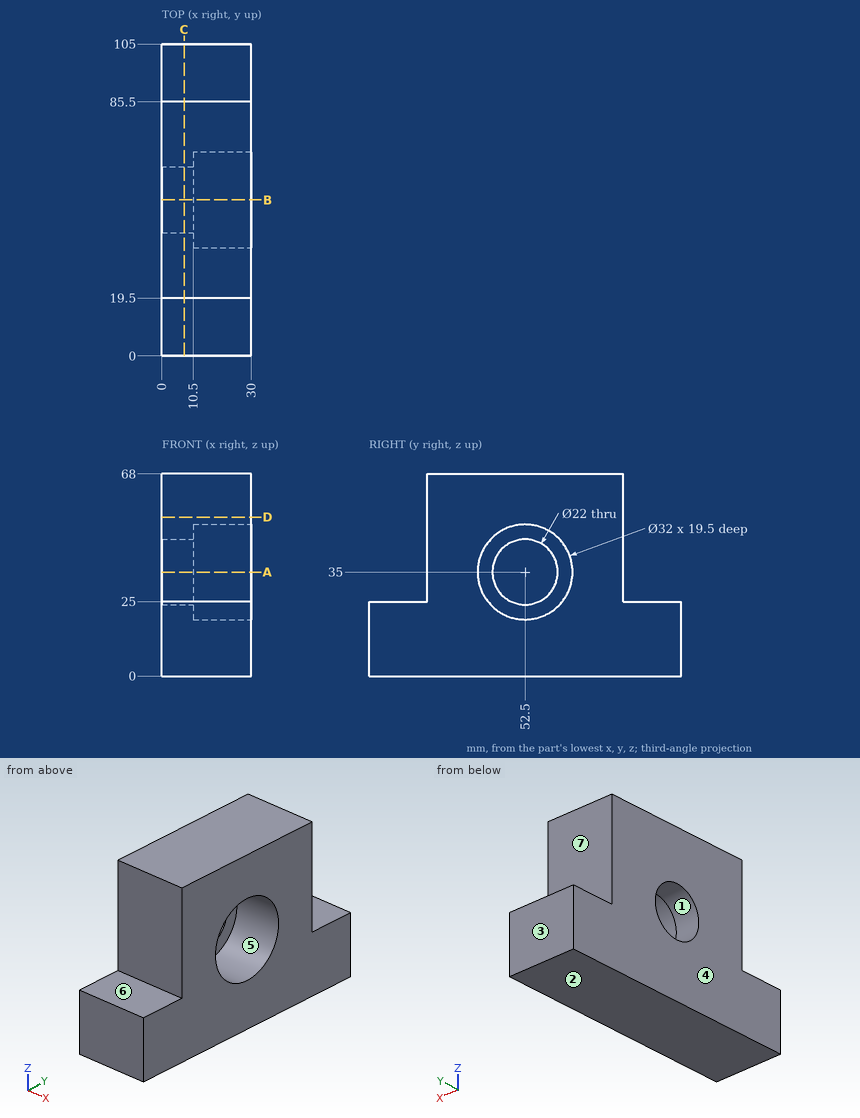
Check sheet for the drawn part. Datum: minimum x, y, z corner. Units: mm. A direction names the side the tool comes from. Give positions to 0.01 mm unless a question says otherwise; leave off trailing zeros. Loops run counter-clockwise (first coordinate to the right, second up) from the corner with the lowest first, then second, coordinate; pieces in that order, holes last.
1) Set-up check for the marked faces 4, 5, 6 and 7: record each of +Z, -Z, +X, -X, +Y, -Y from which the full face is reachable in a straight line by a thin tool's end or side.
2) Sectioned sample at D-D, the plane z = 53.5. Enter the section's corners in (x, y), then the cut area to 3 significant figures.
3) Sectioned sample at C-C, the plane x = 7.5. Enter the section's corners in (y, z).
4) Draft check along Y on the marked faces 1, 2 and 3. Enter one of: pulls with the +Y half, pulls with the -Y half, needs draft (parallel to the pull), parting line crosses it, or undercut.
5) Sectioned sample at A-A, the plane z = 35. Enter the section's corners in (x, y).
6) Sectioned sample at B-B, the plane y = 52.5. Enter the section's corners in (x, z).
7) Depth check by flat-ended pin: pin 1 Ø2 at (x, z) = (3.5, 31.5) entering from +Y; pin 2 Ø17.5 at (y, z) = (52.5, 35) entering from +X; pin 3 Ø9.5 at (y, z) = (46.5, 38) entering from +X; pin 4 Ø2 at (x, z) = (14.5, 46.5) entering from -Y. Enter the tip coordinate at first touch or a pass-through.
8) Thickness scan on line 1 along Z through (x, y) = (8, 52.5); line 2 along Z through (x, y) = (18.5, 52.5); line 3 along X through (y, z) = (37, 32). Record the ranges inside material, lowest first.
Answers:
1. face 4: +Z, -Z, -X, +Y, -Y
1. face 5: +X
1. face 6: +Z, +X, -X, -Y
1. face 7: +Z, +X, -X, +Y
2. outline: (0, 19.5) - (30, 19.5) - (30, 85.5) - (0, 85.5) - close
2. area: 1,980 mm2
3. outline: (0, 0) - (105, 0) - (105, 25) - (85.5, 25) - (85.5, 68) - (19.5, 68) - (19.5, 25) - (0, 25) - close; hole circle Ø22 at (52.5, 35)
4. face 1: undercut
4. face 2: needs draft
4. face 3: pulls with the +Y half
5. outline: (0, 19.5) - (30, 19.5) - (30, 36.5) - (10.5, 36.5) - (10.5, 41.5) - (0, 41.5) - close; (0, 63.5) - (10.5, 63.5) - (10.5, 68.5) - (30, 68.5) - (30, 85.5) - (0, 85.5) - close
6. outline: (0, 0) - (30, 0) - (30, 19) - (10.5, 19) - (10.5, 24) - (0, 24) - close; (0, 46) - (10.5, 46) - (10.5, 51) - (30, 51) - (30, 68) - (0, 68) - close
7. pin 1: stops at y = 85.5
7. pin 2: passes through
7. pin 3: stops at x = 10.5
7. pin 4: stops at y = 19.5
8. line 1: z = 0 to 24, 46 to 68
8. line 2: z = 0 to 19, 51 to 68
8. line 3: x = 0 to 10.5
